Autodesk Inventor part; units mm, degrees
ref_plane "YZ Plane" through (0, 0, 0) normal (1, 0, 0) x (0, 1, 0)
ref_plane "XZ Plane" through (0, 0, 0) normal (0, 1, 0) x (-1, 0, 0)
ref_plane "XY Plane" through (0, 0, 0) normal (0, 0, 1) x (1, 0, 0)
sketch "Sketch3" plane through (0, 0, 0) normal (0, 1, 0) x (-1, 0, 0)
  line L0 (-39.25, 30.5) -> (39.25, 30.5)
  line L1 (39.25, 30.5) -> (39.25, -30.5)
  line L2 (39.25, -30.5) -> (-39.25, -30.5)
  line L3 (-39.25, -30.5) -> (-39.25, 30.5)
  line L4 (-39.25, 30.5) -> (39.25, -30.5) construction
  line L5 (39.25, 30.5) -> (-39.25, -30.5) construction
  point P0 (0, 0)
  dimension "d0" = 78.5
  dimension "d1" = 61
extrude "Extrusion1" add sketch "Sketch3" along normal blind 0.5
sketch "Sketch4" plane through (0, 0.5, 0) normal (0, 1, 0) x (1, 0, 0)
  line L0 (-23.6083, -15) -> (-28.6083, -15)
  line L1 (-28.6083, -15) -> (-28.6083, 15)
  line L2 (-28.6083, 15) -> (-23.6083, 15)
  line L3 (-23.6083, 15) -> (-23.6083, -15)
  line L4 (-23.6083, -15) -> (-28.6083, 15) construction
  line L5 (-28.6083, -15) -> (-23.6083, 15) construction
  point P0 (0, 0)
  point P1 (-26.1083, 0)
  dimension "d4" = 5
  dimension "d5" = 30
extrude "Extrusion2" add sketch "Sketch4" along normal blind 2
fillet "Fillet1" radius 2 4 edges at (-28.6083, 1.5, 15) (-23.6083, 1.5, 15) (-28.6083, 1.5, -15) (-23.6083, 1.5, -15)
fillet "Fillet2" radius 2 4 edges at (-39.25, 0.25, 30.5) (39.25, 0.25, 30.5) (39.25, 0.25, -30.5) (-39.25, 0.25, -30.5)
properties part number "Tutup Pzem test1"
Can you work these out from the model? Positions are in its coordinate system, mm. A direction names the side the tool comes from. Coordinates: 2 decimals unless noted, no trailing zeros. Loops run counter-clockwise (first coordinate to the right, second up) from the corner with the lowest first, then second, coordinate; pieces in that order, holes last. Notation, with made-up numbers: (-19.75, 66) - (-12.75, 66) arc R24 ccw to (-12.75, 94) - close; hole circle Ø3 at (65.5, -13.75). An arc over 180 degrees is marked (long way). Answer as CSV lines item,"result". Start each with the question number.
1) For pin 1 (1 mm diameter, centred on y = 1.5, z = 5, fed in from +X); pin 2 (0.8 mm diameter, centred on x = -26, y = 1.5, fed in from -Z); pin 3 (5 mm diameter, centred on x = 10.5, z = 2, fed in from +Y), each with a flat end and sliding along its axis, tell me the tip position at first contact or that it passes through.
2) Suppose I cut it at D-D (z = 26). Please give me the cut outline in (x, y).
3) Suppose I cut it at A-A (y = 1.25). Please give me the cut outline in (x, z), plus the area to 3 significant figures.
4) Suppose I cut it at B-B (z = 2.5). Please give me the cut outline in (x, y).
5) Which directions (+Z, -Z, +X, -X, +Y, -Y) give clear straight access to the entire face, cutting with the end or side of a thin tool? Please do faces 1 (the cylindrical face through (-24.18, 1.51, -14.4)), 2 (the flat face through (-28.608, 1, 0)), 3 (the flat face through (-23.608, 1, 0)), 4 (the cylindrical face through (-24.21, 1.51, 14.43)), 5 (the cylindrical face through (-28.038, 1.514, 14.399)).
6) Suppose I cut it at C-C (x = 33). Please give me the cut outline in (y, z).
7) I need wall thicknesses on line 1 (X direction, y = 2.2, z = -9); line 2 (Y direction, x = -3, z = 26); line 3 (X direction, y = 1.9, z = 13.5). Which ranges of each line are inside material? Lowest first, please. Write a range as from..to.
Check result:
1,pin 1,"stops at x = -23.61"
1,pin 2,"stops at z = -15"
1,pin 3,"stops at y = 0.5"
2,outline,"(-39.25, 0) - (39.25, 0) - (39.25, 0.5) - (-39.25, 0.5) - close"
3,outline,"(-28.61, -13) arc R2 ccw to (-26.61, -15) - (-25.61, -15) arc R2 ccw to (-23.61, -13) - (-23.61, 13) arc R2 ccw to (-25.61, 15) - (-26.61, 15) arc R2 ccw to (-28.61, 13) - close"
3,area,"147 mm²"
4,outline,"(-39.25, 0) - (39.25, 0) - (39.25, 0.5) - (-23.61, 0.5) - (-23.61, 2.5) - (-28.61, 2.5) - (-28.61, 0.5) - (-39.25, 0.5) - close"
5,face 1,"-Z, +X, +Y"
5,face 2,"+Z, -Z, -X, +Y"
5,face 3,"+Z, -Z, +X, +Y"
5,face 4,"+Z, +X, +Y"
5,face 5,"+Z, -X, +Y"
6,outline,"(0, -30.5) - (0.5, -30.5) - (0.5, 30.5) - (0, 30.5) - close"
7,line 1,"x = -28.61..-23.61"
7,line 2,"y = 0..0.5"
7,line 3,"x = -28.54..-23.67"
